```python
from build123d import *

# Parameters (mm, degrees)
EXTRUDE_1_DEPTH     = 3.2
SKETCH_2_R          = 2
CUT_EXTRUDE_1_DEPTH = 3.2
FILLET_1_R          = 0.16


with BuildPart() as part:
    # 草图1 → 凸台-拉伸1 (new body)
    with BuildSketch(Plane.XY):
        Polygon((0, 4.041451884), (-3.5, 2.020725942), (-3.5, -2.020725942), (0, -4.041451884), (3.5, -2.020725942), (3.5, 2.020725942), align=None)
    extrude(amount=EXTRUDE_1_DEPTH)

    # 草图2 → 切除-拉伸1 (cut)
    with BuildSketch(Plane(origin=(0, 0, 0), x_dir=(-1, 0, 0), z_dir=(0, 0, -1))):
        Circle(SKETCH_2_R)
    extrude(amount=-CUT_EXTRUDE_1_DEPTH, mode=Mode.SUBTRACT)

    # 草图4 → 切除-旋转1 (revolve, cut)
    with BuildSketch(Plane(origin=(0, 0, 0), x_dir=(0, 0, -1), z_dir=(1, 0, 0))):
        Polygon((-2.677, 4.041451884), (-3.2, 3.518451884), (-3.2, 4.041451884), align=None)
        Polygon((0, 4.041451884), (-0.523, 4.041451884), (0, 3.518451884), align=None)
    revolve(axis=Axis((0, 0, 0), (0, 0, 1)), mode=Mode.SUBTRACT)

    # 圆角1
    fillet_1_edges = [part.edges().sort_by_distance(p)[0] for p in [
        (2, 0, 3.2),
        (2, 0, 0),
    ]]
    fillet(fillet_1_edges, radius=FILLET_1_R)


solid = part.part
```
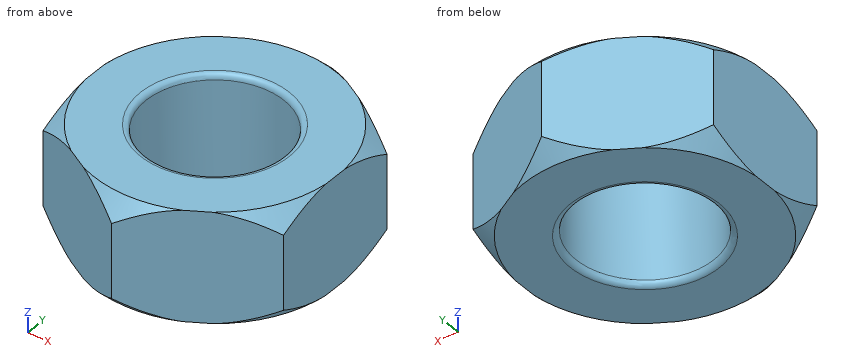
Work out the finished part from the listing and answer in its coordinate system (mm). Coordinates: 2 decimals unless noted, no trailing zeros. Order: outer loops, then holes, each group sorted by start corner. A loop starts at its lowest first (then second) coordinate and runs counter-clockwise, first axis right, second up. Notation, with made-up numbers: M -10.5,-17.5 L 12.5,-17.5 A12 cw 12.5,0.5 Z; hole C 26,78 d9. An arc over 180 degrees is marked long. Use CSV: the item, a comma, the result in double quotes.
1) Section B-B on y = 0 is taken. Write down the section's boundary in (x, z), plus the area to 3 significant figures.
Worked out:
outline,"M -3.5,0 L -2.16,0 A0.16 ccw -2,0.16 L -2,3.04 A0.16 ccw -2.16,3.2 L -3.5,3.2 Z; M 2,0.16 A0.16 ccw 2.16,0 L 3.5,0 L 3.5,3.2 L 2.16,3.2 A0.16 ccw 2,3.04 Z"
area,"9.58 mm^2"
2) Section A-A on z = 2.2 is taken. Write down the section's boundary in (x, y), plus the area to 3 significant figures.
Worked out:
outline,"M -3.5,-2.02 L 0,-4.04 L 3.5,-2.02 L 3.5,2.02 L 0,4.04 L -3.5,2.02 Z; hole C 0,0 d4"
area,"29.9 mm^2"
3) Section D-D on y = 3 is taken. Write down the section's boundary in (x, z).
Worked out:
outline,"M -1.8,0 L 1.8,0 L 1.8,3.2 L -1.8,3.2 Z"
4) Section C-C on z = 2.95 is taken. Write down the section's boundary in (x, y).
Worked out:
outline,"M -3.5,-1.4 A3.77 ccw -2.96,-2.33 L -0.54,-3.73 A3.77 ccw 0.54,-3.73 L 2.96,-2.33 A3.77 ccw 3.5,-1.4 L 3.5,1.4 A3.77 ccw 2.96,2.33 L 0.54,3.73 A3.77 ccw -0.54,3.73 L -2.96,2.33 A3.77 ccw -3.5,1.4 Z; hole C 0,0 d4"
5) Consider line 1 (X direction, y = 0.5, z = 2.7); line 2 (Y direction, x = -1, z = 1.5); line 3 (Y direction, x = -1.25, z = 0.8). Determine where each line is inside the solid, lowest interval first. Write a range as [from, to].
Worked out:
line 1,"x = [-3.5, -1.94], [1.94, 3.5]"
line 2,"y = [-3.46, -1.73], [1.73, 3.46]"
line 3,"y = [-3.32, -1.56], [1.56, 3.32]"
